Design review of the part built by this model. Coordinates are the model's own, in mm. Face numbers are marked on the shaded views. A direction names the side the tool comes from. Coordinates: 2 decimals unless noted, no trailing zeros. Order: outer loops, then holes, each group sorted by start corner. A loop starts at its lowest first (then second) coordinate and runs counter-clockwise, first axis right, second up. Notation, with made-up numbers: M -33,-3 L 25,-3 A22 ccw 25,33 Z; hole C -4,42 d6. An arc over 180 degrees is marked long. Answer as a JSON object with one key per item and string values.
from build123d import *

# Parameters (mm, degrees)
F0_W     = 91.255646
F0_H     = 38.714515
F1_DEPTH = 14.732
F2_W     = 51.619354
F2_H     = 29.128062
F3_DEPTH = 8.636
F4_R     = 2.219926
F5_DEPTH = 2.794
F7_DEPTH = 10.668
F8_R     = 6.600831
F9_DEPTH = 25.4


with BuildPart() as f1:
    # F0 (on Front) → F1 (new body)
    with BuildSketch(Plane.XZ):
        with Locations((7.005485, -3.410563)):
            Rectangle(F0_W, F0_H)
    extrude(amount=F1_DEPTH)

    # F2 (on face) → F3 (cut)
    with BuildSketch(Plane.XZ.offset(14.732)):
        with Locations((2.857499, -3.22621)):
            Rectangle(F2_W, F2_H)
    extrude(amount=-F3_DEPTH, mode=Mode.SUBTRACT)

    # F4 (on face) → F5 (cut)
    with BuildSketch(Plane.XZ.offset(6.096)):
        with Locations((-15.946694, -2.48879)):
            Circle(F4_R)
    extrude(amount=-F5_DEPTH, mode=Mode.SUBTRACT)

    # F6 (on face) → F7 (cut)
    with BuildSketch(Plane.XZ.offset(14.732)):
        with BuildLine():
            Line((33.276051, 0), (33.276051, -3.22621))
            Line((33.276051, -3.22621), (33.276051, -7.466371))
            Line((33.276051, -7.466371), (40.465884, -7.466371))
            ThreePointArc((40.465884, -7.466371), (44.199069, -3.733185), (40.465884, 0))
            Line((40.465884, 0), (33.276051, 0))
        make_face()
    extrude(amount=-F7_DEPTH, mode=Mode.SUBTRACT)

    # F8 (on face) → F9 (join)
    with BuildSketch(Plane.XZ.offset(6.096)):
        with Locations((10.969113, -1.567016)):
            Circle(F8_R)
    extrude(amount=F9_DEPTH)


solid = f1.part
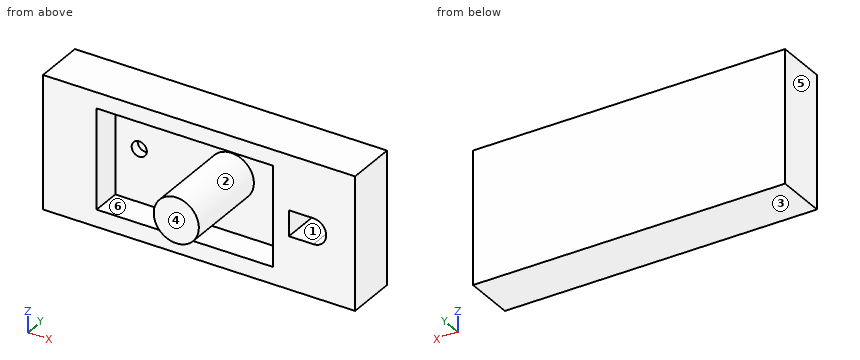
1) To check wall thickness, follow L1, parallel to Z at x = 28, y = -13; L2, parallel to X at y = -13.5, z = -8.5; L3, parallel to X at y = -10, z = -3.5. State the ranges of each line that lie inside material, in increasing order.
Taken from the geometry:
{"L1": "z = -22.77 to -17.79, 11.34 to 15.95", "L2": "x = -38.62 to -22.95, 28.67 to 52.63", "L3": "x = -38.62 to -22.95, 4.66 to 17.28, 28.67 to 33.28, 44.19 to 52.63"}
2) Add section B-B (z = -13). State the section outline as (x, y) points.
Taken from the geometry:
{"outline": "M -38.62,-14.73 L -22.95,-14.73 L -22.95,-6.1 L 28.67,-6.1 L 28.67,-14.73 L 52.63,-14.73 L 52.63,0 L -38.62,0 Z"}
3) Mouldability with a two-part tool opening along Z and no side actions: class the marked faces 1, 2, 3 and 4 as released by +Z, released by -Z, zero draft, split by the parting line, or undercut.
Taken from the geometry:
{"face 1": "undercut", "face 2": "undercut", "face 3": "released by -Z", "face 4": "zero draft"}
4) Tool access review of the marked faces 5 and 6: name each direction out of +Z, -Z, +X, -X, +Y, -Y from which nothing blocks a thin tool from reaching the whole face with its end or side.
Taken from the geometry:
{"face 5": "+Z, -Z, -X, +Y, -Y", "face 6": "-Y"}
5) Add section C-C (x = -10). State the section outline as (y, z) points, and give its area (3 significant figures).
Taken from the geometry:
{"outline": "M -14.73,-22.77 L 0,-22.77 L 0,15.95 L -14.73,15.95 L -14.73,11.34 L -6.1,11.34 L -6.1,-17.79 L -14.73,-17.79 Z", "area": "319 mm2"}
6) Add section A-A (y = -9.5). State the section outline as (x, z) points, and give its area (3 significant figures).
Taken from the geometry:
{"outline": "M -38.62,-22.77 L 52.63,-22.77 L 52.63,15.95 L -38.62,15.95 Z; C 10.97,-1.57 d13.2; hole M -22.95,-17.79 L 28.67,-17.79 L 28.67,11.34 L -22.95,11.34 Z; hole M 33.28,-7.47 L 40.47,-7.47 A3.73 ccw 40.47,0 L 33.28,0 Z", "area": "2,090 mm2"}
7) Add section D-D (z = 3.5). State the section outline as (x, y) points, and give its area (3 significant figures).
Taken from the geometry:
{"outline": "M -38.62,-14.73 L -22.95,-14.73 L -22.95,-6.1 L 6.74,-6.1 L 6.74,-31.5 L 15.2,-31.5 L 15.2,-6.1 L 28.67,-6.1 L 28.67,-14.73 L 52.63,-14.73 L 52.63,0 L -38.62,0 Z", "area": "1,110 mm2"}
8) Insertion check: pin 1 Ø6 at (x, z) = (-15.95, -2.49) entering from -Y; pin 2 Ø10 at (x, z) = (24.5, 6) entering from -Y; pin 3 Ø4 at (y, z) = (-17, 8.5) entering from -X; pin 4 Ø10 at (y, z) = (-22.5, 8) entering from +X. Each pin has a flat end and moves straight along its axis. Give the tip position at first contact, or say it passes through.
Taken from the geometry:
{"pin 1": "stops at y = -6.1", "pin 2": "stops at y = -14.73", "pin 3": "passes through", "pin 4": "stops at x = 15.73"}
